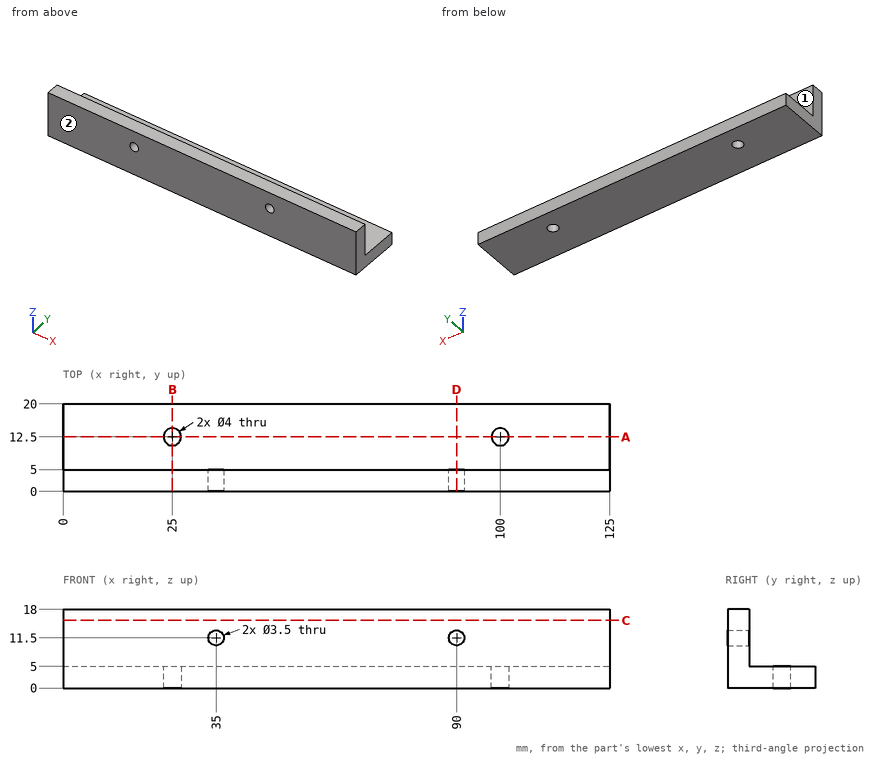
Source: three-view drawing plus pictorial views. Frame: mm from the lowest corner of the part. A direction names the side the tool comes from. Give positions to 0.01 mm unless a question says otherwise; leave off trailing zeros. Order: outer loops, then holes, each group sorted by start corner. A loop starts at its lowest first (then second) coordinate and runs counter-clockwise, first axis right, second up.
1. Reachability of the marked faces 1 and 2 from +Z, -Z, +X, -X, +Y, -Y: full face, straight path, thin tool, end or side. Return the list, or none.
Derived:
face 1: +Z, +X, -X, +Y
face 2: +Z, -Z, +X, -X, -Y
2. Section D-D on x = 90. Return the cut outline in (y, z), and give its area (4 significant figures).
Derived:
outline: (0, 0) - (20, 0) - (20, 5) - (5, 5) - (5, 9.75) - (0, 9.75) - close; (0, 13.25) - (5, 13.25) - (5, 18) - (0, 18) - close
area: 147.5 mm2
3. Pin query (flat end, axial travel): pin 1 (4.5 mm diameter, centred on x = 90, z = 11.5, fed in from +Y); pin 2 (3 mm diameter, centred on x = 25, y = 12.5, fed in from +Z); pin 3 (6 mm diameter, centred on x = 38, y = 14, fed in from +Z). Return the tip coordinate at first contact, or that it passes through.
Derived:
pin 1: stops at y = 5
pin 2: passes through
pin 3: stops at z = 5
4. Section A-A on y = 12.5. Return the cut outline in (x, z).
Derived:
outline: (0, 0) - (23, 0) - (23, 5) - (0, 5) - close; (27, 0) - (98, 0) - (98, 5) - (27, 5) - close; (102, 0) - (125, 0) - (125, 5) - (102, 5) - close
5. Material intervals for L1, parallel to X at y = 1.45, z = 11.5; L2, parallel to Z at x = 90, y = 2.6; L3, parallel to Y at x = 108, z = 15, sorted ascending.
Derived:
L1: x = 0 to 33.25, 36.75 to 88.25, 91.75 to 125
L2: z = 0 to 9.75, 13.25 to 18
L3: y = 0 to 5
6. Section C-C on z = 15.5. Return the cut outline in (x, y), and give its area (3 significant figures).
Derived:
outline: (0, 0) - (125, 0) - (125, 5) - (0, 5) - close
area: 625 mm2
7. Section B-B on x = 25. Return the cut outline in (y, z), and give its area (3 significant figures).
Derived:
outline: (0, 0) - (10.5, 0) - (10.5, 5) - (5, 5) - (5, 18) - (0, 18) - close; (14.5, 0) - (20, 0) - (20, 5) - (14.5, 5) - close
area: 145 mm2
